Autodesk Fusion 360 part; units mm, degrees
sketch "Sketch1" plane through (0, 0, 0) normal (0, 1, 0) x (1, 0, 0)
  circle A0 centre (0, 0) radius 70
  dimension "d1" = 140
extrude "Extrude1" add sketch "Sketch1" along normal blind 10
sketch "Sketch2" plane through (0, 0, 0) normal (0, -1, 0) x (1, 0, 0)
  circle A0 centre (0, 0) radius 70
  circle A1 centre (0, 0) radius 65
  dimension "d4" = -5
extrude "Extrude2" add sketch "Sketch2" along normal blind 3 contours A1
sketch "Sketch3" plane through (0, 0, 0) normal (0, 0, 1) x (1, 0, 0)
  line L0 (-25, 55) -> (-25, 5)
  line L1 (-25, 5) -> (-90, 5)
  line L2 (-90, 5) -> (-102.7928, 41.8964)
  arc A0 (-25, 55) -> (-102.7928, 41.8964) centre (-65, 55) ccw
  dimension "d7" = 50
  dimension "d8" = 65
  dimension "d9" = 40
  dimension "d10" = 5
  dimension "d11" = 25
extrude "Extrude3" add sketch "Sketch3" along normal mid plane 10
sketch "Sketch4" plane through (0, 10, 0) normal (0, 1, 0) x (-1, 0, 0)
  line L0 (25, 5) -> (69.8212, 5)
  arc A0 (69.8212, 5) -> (69.8212, -5) centre (0, 0) ccw
  line L1 (69.8212, -5) -> (25, -5)
  line L2 (25, -5) -> (25, 5)
  line L3 (-6.378, -23.622) -> (-53.622, -23.622)
  line L4 (-53.622, -23.622) -> (-53.622, 23.622)
  line L5 (-53.622, 23.622) -> (-6.378, 23.622)
  line L6 (-6.378, 23.622) -> (-6.378, -23.622)
  line L7 (-6.378, -23.622) -> (-53.622, 23.622) construction
  line L8 (-53.622, -23.622) -> (-6.378, 23.622) construction
  point P0 (-30, 0)
  dimension "d14" = 47.244
  dimension "d15" = 47.244
  dimension "d16" = 30
hole "Hole1" at (6.378, 10, 23.622) at (6.378, 10, -23.622) at (53.622, 10, -23.622) at (53.622, 10, 23.622) direction (0, -1, 0) diameter 4 depth 10 tip angle 118
hole "Hole2" at (30, 10, 0) direction (0, -1, 0) diameter 6 depth 15 tip angle 118
sketch "Sketch5" plane through (0, 0, 5) normal (0, 0, 1) x (1, 0, 0)
  line L0 (-69.8212, 10) -> (-25, 10)
  line L1 (-25, 10) -> (-25, 55)
  arc A0 (-25, 55) -> (-102.7928, 41.8964) centre (-65, 55) ccw
  line L2 (-102.7928, 41.8964) -> (-90, 5)
  line L3 (-90, 5) -> (-69.8212, 5)
  line L4 (-69.8212, 5) -> (-69.8212, 10)
  line L5 (-41.378, 78.622) -> (-88.622, 78.622)
  line L6 (-88.622, 78.622) -> (-88.622, 31.378)
  line L7 (-88.622, 31.378) -> (-41.378, 31.378)
  line L8 (-41.378, 31.378) -> (-41.378, 78.622)
  line L9 (-41.378, 78.622) -> (-88.622, 31.378) construction
  line L10 (-88.622, 78.622) -> (-41.378, 31.378) construction
  point P0 (-65, 55)
  dimension "d23" = 47.244
  dimension "d24" = 47.244
hole "Hole3" at (-88.622, 78.622, 5) at (-41.378, 78.622, 5) at (-41.378, 31.378, 5) at (-88.622, 31.378, 5) direction (0, 0, -1) diameter 4 depth 40 tip angle 118
hole "Hole4" at (-65, 55, 5) direction (0, 0, -1) diameter 6 depth 40 tip angle 118
Geometry: final body of the model. Coordinates: model frame, mm. A direction names the side the tool comes from. Round coordinates to 2 decimals unless told otherwise and drop trailing zeros. Order: outer loops, then holes, each group sorted by start corner. A loop starts at its lowest first (then second) coordinate and runs counter-clockwise, first axis right, second up. Notation, with made-up numbers: M 73.5,-34.75 L 95.5,-34.75 A10 ccw 95.5,-25.75 Z; hole C 87,-1.75 d3. An arc over 180 degrees is marked long. Use one line per item in the form item = value. Start each with the question number.
Q1. Cut plane A-A (z = 0). Return loops of the section in (x, y).
Q2. Material intervals for line 1 (Y direction, x = -41.5, z = 0.5); line 2 (Y direction, x = -33, z = -42); line 3 (X direction, y = 9.5, z = 24), sorted ascending. Write a range as [from, to].
Q3. Cut plane B-B (x = 30). Return loops of the section in (y, z), and give its area (3 significant figures).
Q4. Cut plane D-D (z = 14). Return loops of the section in (x, y), and give its area (3 significant figures).
Q5. Pin query (flat end, axial travel): pin 1 Ø4.5 at (x, y) = (-41.378, 78.622) entering from +Z; pin 2 Ø8 at (x, z) = (30, 0) entering from +Y; pin 3 Ø11 at (y, z) = (29, -0.5) entering from +X. Return the tip coordinate at first contact, or that it passes through.
Q6. Mould query, pull axis Y, two halves, no side actions, for faces 1 (the face through (-63.2, 57.4, -0.1)), 2 (the face through (-25, 33, 0)), 3 (the face through (53.97, -0.99, -23.67)). Classes: +Y half, -Y half, draft (parallel to the pull), parting line (faces both ways), or undercut.
Q7. Access query for faces 4 (the face through (-80, 5, 0)), 5 (the face through (61.9, 0, 20.4)), 6 (the face through (7.59, 4.93, 22.03)). Directions: +Z, -Z, +X, -X, +Y, -Y. A direction counts if a zero-diameter tool reaches every point of the face in a straight line with its end or side. Return the directions, or none.
Q8. Cut plane C-C (x = 0). Return loops of the section in (y, z).
Geometry results:
q1.outline = M -102.79,41.9 L -90,5 L -70,5 L -70,0 L -65,0 L -65,-3 L 27,-3 L 27,10 L -25,10 L -25,55 A40 ccw long Z; M 33,-3 L 65,-3 L 65,0 L 70,0 L 70,10 L 33,10 Z; hole C -88.62,31.38 d4; hole C -88.62,78.62 d4; hole C -65,55 d6; hole C -41.38,31.38 d4; hole C -41.38,78.62 d4
q2.line_1 = [-3, 29.38], [33.37, 76.63], [80.62, 87.37]
q2.line_2 = [-3, 10]
q2.line_3 = [-65.76, 4.41], [8.34, 51.66], [55.59, 65.76]
q3.outline = M -3,-57.66 L 0,-57.66 L 0,-63.25 L 10,-63.25 L 10,-3 L -3,-3 Z; M -3,3 L 10,3 L 10,63.25 L 0,63.25 L 0,57.66 L -3,57.66 Z
q3.area = 1,530 mm^2
q4.outline = M -68.59,0 L -63.47,0 L -63.47,-3 L 63.47,-3 L 63.47,0 L 68.59,0 L 68.59,10 L -68.59,10 Z
q4.area = 1,750 mm^2
q5.pin_1 = 5
q5.pin_2 = 10
q5.pin_3 = -25
q6.face_1 = undercut
q6.face_2 = draft
q6.face_3 = +Y half
q7.face_4 = +Z, -Z, -X, -Y
q7.face_5 = -Y
q7.face_6 = +Y
q8.outline = M -3,-65 L 0,-65 L 0,-70 L 10,-70 L 10,70 L 0,70 L 0,65 L -3,65 Z
